Can you work these out from the drawing? Everything is in mm from the part's minimum corner. Give positions to 0.01 mm unless a question says otherwise; leave off trailing zeros. Write each loop counter-clockwise with the first axis right and the second up, starting at its lowest first coordinate (ties: lowest second). Pieces come first, ordered by that corner, then holes. Notation, with made-up numbers: (71.5, -10.75) -> (121.5, -10.75) arc R21 ccw to (121.5, 25.25) -> close; hole circle Ø5 at (84.5, -27.5). An arc over 180 degrees is marked (long way). Answer as CSV lines item,"result". Start each with the question number.
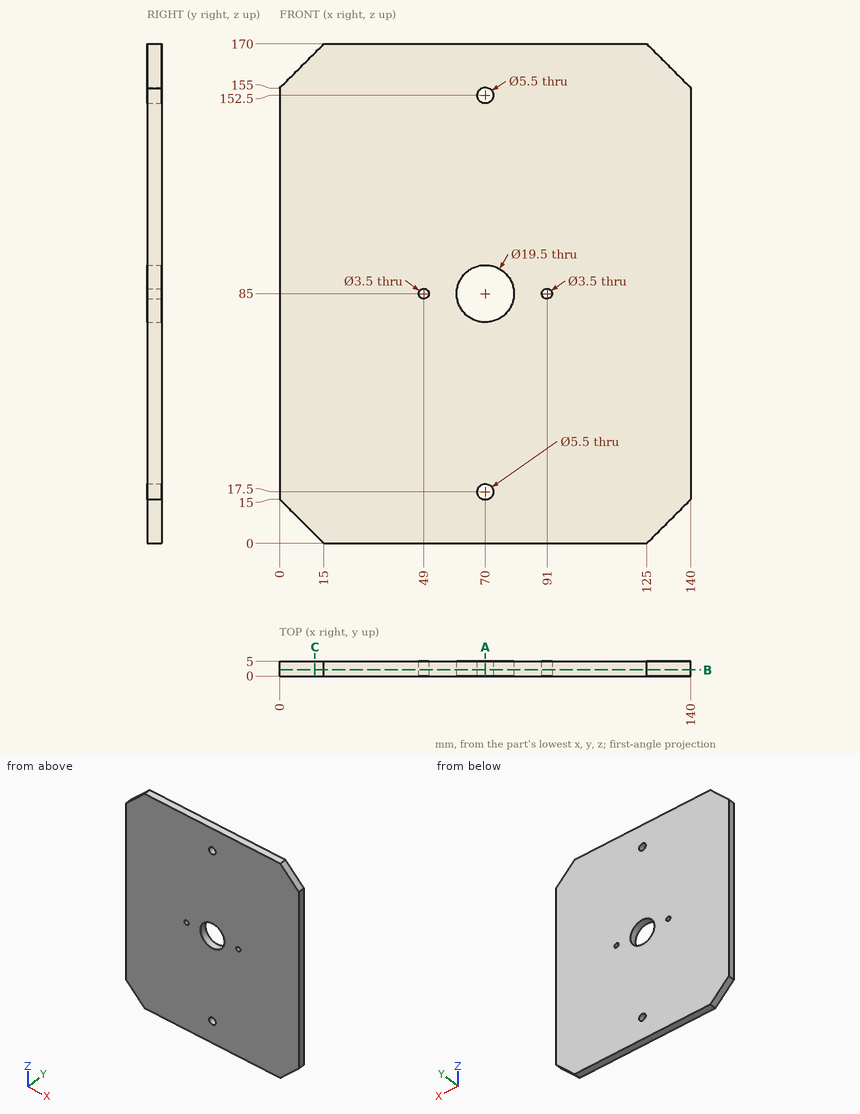
Item 1: If I drill on line 1 (X direction, y = 3.9, z = 85); line 2 (Z direction, x = 70, y = 1.55); line 3 (Z direction, x = 49, y = 2.5), over which ranges is the centre line in solid material (lowest first)? Write a range as [from, to].
Item 2: If we section it at B-B (y = 2.05): Please give me the cut outline in (x, z).
Item 3: I'm going to push a flat-ended pin straight in: pin 1 (3 mm diameter, centred on x = 49, z = 85, fed in from -Y). Where does the tip first touch, or does it pass through?
Item 4: If we section it at A-A (x = 70): Please give me the cut outline in (y, z), and give its area (4 significant figures).
Item 5: If we section it at C-C (x = 12): Please give me the cut outline in (y, z), and give its area (3 significant figures).
Final values:
1,line 1,"[0, 47.25], [50.75, 60.25], [79.75, 89.25], [92.75, 140]"
1,line 2,"[0, 14.75], [20.25, 75.25], [94.75, 149.75], [155.25, 170]"
1,line 3,"[0, 83.25], [86.75, 170]"
2,outline,"(0, 15) -> (15, 0) -> (125, 0) -> (140, 15) -> (140, 155) -> (125, 170) -> (15, 170) -> (0, 155) -> close; hole circle Ø3.5 at (49, 85); hole circle Ø19.5 at (70, 85); hole circle Ø5.5 at (70, 17.5); hole circle Ø5.5 at (70, 152.5); hole circle Ø3.5 at (91, 85)"
3,pin 1,"through"
4,outline,"(0, 0) -> (5, 0) -> (5, 14.75) -> (0, 14.75) -> close; (0, 20.25) -> (5, 20.25) -> (5, 75.25) -> (0, 75.25) -> close; (0, 94.75) -> (5, 94.75) -> (5, 149.75) -> (0, 149.75) -> close; (0, 155.25) -> (5, 155.25) -> (5, 170) -> (0, 170) -> close"
4,area,"697.5 mm2"
5,outline,"(0, 3) -> (5, 3) -> (5, 167) -> (0, 167) -> close"
5,area,"820 mm2"
